```python
from build123d import *

# Parameters (mm, degrees)
F0_W      = 146.1516
F0_H      = 143.1798
F1_DEPTH  = 20.9042
F2_W      = 136.906
F2_H      = 134.874
F3_DEPTH  = 12.7
F4_W      = 13.97
F4_H      = 11.176
F5_DEPTH  = 12.7
F6_W      = 22.733
F6_H      = 6.096
F7_DEPTH  = 12.7
F8_W      = 15.367
F8_H      = 5.08
F9_DEPTH  = 12.7
F10_W     = 36.703
F10_H     = 12.319
F11_DEPTH = 12.7
F13_DEPTH = 12.7
F14_W     = 22.83968
F14_H     = 21.22805
F15_DEPTH = 12.7
F16_W     = 3.0399242607
F16_H     = 20.8479667597
F17_DEPTH = 12.7
F19_DEPTH = 12.7
F20_W     = 0.0204666441
F20_H     = 21.22805
F21_DEPTH = 12.7
F22_W     = 36.7188937962
F22_H     = 20.8685005598
F23_DEPTH = 12.7
F24_W     = 35.306
F24_H     = 13.2634267211
F25_DEPTH = 12.7
F27_DEPTH = 12.7
F28_W     = 1.4742958935
F28_H     = 20.8479667597
F29_DEPTH = 12.7
F30_W     = 0.2049181255
F30_H     = 13.2839605212
F31_DEPTH = 12.7
F32_W     = 50.9417812916
F32_H     = 3.8105603307
F33_DEPTH = 12.7
F34_W     = 0.1417576911
F34_H     = 9.2577636242
F35_DEPTH = 12.7
F36_W     = 44.7041876614
F36_H     = 0.2025440335
F37_DEPTH = 12.7
F38_W     = 8.9374343662
F38_H     = 3.9174016565
F39_DEPTH = 12.7
F40_W     = 127.9685656338
F40_H     = 2.8044246137
F41_DEPTH = 12.7
F42_W     = 120.384439826
F42_H     = 1.1129770428
F43_DEPTH = 12.7
F45_DEPTH = 12.7
F46_W     = 12.3281155104
F46_H     = 3.9624
F47_DEPTH = 12.7
F48_W     = 4.6508648958
F48_H     = 7.4722463233
F49_DEPTH = 12.7
F51_DEPTH = 12.7
F52_W     = 0.5965952
F52_H     = 1.6107708216
F53_DEPTH = 12.7
F55_DEPTH = 12.7
F57_DEPTH = 12.7
F58_DEPTH = 12.7
F59_W     = 18.6266698875
F59_H     = 19.8514753814
F60_DEPTH = 12.7
F61_W     = 2.536320244
F61_H     = 7.62
F62_DEPTH = 12.7


with BuildPart() as f1:
    # F0 (on Top) → F1 (new body)
    with BuildSketch(Plane.XY):
        Rectangle(F0_W, F0_H)
    extrude(amount=F1_DEPTH)

    # F2 (on face) → F3 (cut)
    with BuildSketch(Plane.XY.offset(20.9042)):
        Rectangle(F2_W, F2_H)
    extrude(amount=-F3_DEPTH, mode=Mode.SUBTRACT)

    # F4 (on face) → F5 (join)
    with BuildSketch(Plane.XY.offset(8.2042)):
        with Locations((-61.468, -61.849)):
            Rectangle(F4_W, F4_H)
    extrude(amount=F5_DEPTH)

    # F6 (on face) → F7 (join)
    with BuildSketch(Plane.XY.offset(8.2042)):
        with Locations((-43.1165, -59.309)):
            Rectangle(F6_W, F6_H)
    extrude(amount=F7_DEPTH)

    # F8 (on face) → F9 (join)
    with BuildSketch(Plane.XY.offset(8.2042)):
        with Locations((-39.4335, -64.897)):
            Rectangle(F8_W, F8_H)
    extrude(amount=F9_DEPTH)

    # F10 (on face) → F11 (join)
    with BuildSketch(Plane.XY.offset(8.2042)):
        with Locations((50.1015, -61.2775)):
            Rectangle(F10_W, F10_H)
    extrude(amount=F11_DEPTH)

    # F12 (on face) → F13 (join)
    with BuildSketch(Plane.XY.offset(8.2042)):
        Polygon((31.75, -56.261), (31.75, -55.118), (-60.8972720802, -55.118), (-60.8972720802, -56.261), (-31.75, -56.261), (-31.75, -59.817), (31.75, -59.817), (31.75, -57.820610702), align=None)
    extrude(amount=F13_DEPTH)

    # F14 (on face) → F15 (join)
    with BuildSketch(Plane.XY.offset(8.2042)):
        with Locations((-12.7041547344, -44.503975)):
            Rectangle(F14_W, F14_H)
    extrude(amount=F15_DEPTH)

    # F16 (on face) → F17 (join)
    with BuildSketch(Plane.XY.offset(8.2042)):
        with Locations((0.235647396, -44.6940166202)):
            Rectangle(F16_W, F16_H)
    extrude(amount=F17_DEPTH)

    # F18 (on face) → F19 (join)
    with BuildSketch(Plane.XY.offset(8.2042)):
        Polygon((24.1150483489, -33.88995), (1.2599385809, -33.88995), (1.2599385809, -34.2700332403), (1.7556095263, -34.2700332403), (1.7556095263, -55.118), (24.1150483489, -55.118), align=None)
    extrude(amount=F19_DEPTH)

    # F20 (on face) → F21 (join)
    with BuildSketch(Plane.XY.offset(8.2042)):
        with Locations((-24.1342280564, -44.503975)):
            Rectangle(F20_W, F20_H)
    extrude(amount=F21_DEPTH)

    # F22 (on face) → F23 (join)
    with BuildSketch(Plane.XY.offset(8.2042)):
        with Locations((42.474495247, -44.6837497201)):
            Rectangle(F22_W, F22_H)
    extrude(amount=F23_DEPTH)

    # F24 (on face) → F25 (join)
    with BuildSketch(Plane.XY.offset(8.2042)):
        with Locations((43.1809421451, -27.6177860796)):
            Rectangle(F24_W, F24_H)
    extrude(amount=F25_DEPTH)

    # F26 (on face) → F27 (join)
    with BuildSketch(Plane.XY.offset(8.2042)):
        Polygon((-25.618757272, -20.9860727191), (-60.924757272, -20.9860727191), (-60.924757272, -55.118), (-60.8972720802, -55.118), (-25.618757272, -55.118), align=None)
    extrude(amount=F27_DEPTH)

    # F28 (on face) → F29 (join)
    with BuildSketch(Plane.XY.offset(8.2042)):
        with Locations((-24.8816093252, -44.6940166202)):
            Rectangle(F28_W, F28_H)
    extrude(amount=F29_DEPTH)

    # F30 (on face) → F31 (join)
    with BuildSketch(Plane.XY.offset(8.2042)):
        with Locations((-25.5162982092, -27.6280529797)):
            Rectangle(F30_W, F30_H)
    extrude(amount=F31_DEPTH)

    # F32 (on face) → F33 (join)
    with BuildSketch(Plane.XY.offset(8.2042)):
        with Locations((0.0570514993, -22.8913528845)):
            Rectangle(F32_W, F32_H)
    extrude(amount=F33_DEPTH)

    # F34 (on face) → F35 (join)
    with BuildSketch(Plane.XY.offset(8.2042)):
        with Locations((25.4570632995, -29.6206176281)):
            Rectangle(F34_W, F34_H)
        Polygon((25.5279421451, -24.991735816), (25.5279421451, -24.7966330498), (21.3277284056, -24.7966330498), (21.3277284056, -24.991735816), (25.386184454, -24.991735816), align=None)
    extrude(amount=F35_DEPTH)

    # F36 (on face) → F37 (join)
    with BuildSketch(Plane.XY.offset(8.2042)):
        with Locations((-3.0617453158, -24.8979050666)):
            Rectangle(F36_W, F36_H)
    extrude(amount=F37_DEPTH)

    # F38 (on face) → F39 (join)
    with BuildSketch(Plane.XY.offset(8.2042)):
        with Locations((-63.9842828169, 21.8571154401)):
            Rectangle(F38_W, F38_H)
    extrude(amount=F39_DEPTH)

    # F40 (on face) → F41 (join)
    with BuildSketch(Plane.XY.offset(8.2042)):
        with Locations((4.4687171831, 22.4136039615)):
            Rectangle(F40_W, F40_H)
    extrude(amount=F41_DEPTH)

    # F42 (on face) → F43 (join)
    with BuildSketch(Plane.XY.offset(8.2042)):
        with Locations((0.6766542792, 20.4549031332)):
            Rectangle(F42_W, F42_H)
    extrude(amount=F43_DEPTH)

    # F44 (on face) → F45 (join)
    with BuildSketch(Plane.XY.offset(8.2042)):
        Polygon((-60.924757272, 19.8984146118), (-60.924757272, -20.9860727191), (60.8339421451, -20.9860727191), (60.8688741922, -20.9860727191), (60.8688741922, 19.8984146118), align=None)
    extrude(amount=F45_DEPTH)

    # F46 (on face) → F47 (join)
    with BuildSketch(Plane.XY.offset(8.2042)):
        with Locations((-62.2889422448, 33.2692625916)):
            Rectangle(F46_W, F46_H)
    extrude(amount=F47_DEPTH)

    # F48 (on face) → F49 (join)
    with BuildSketch(Plane.XY.offset(8.2042)):
        Polygon((-59.9482320249, 47.5855246186), (-56.1248844896, 47.5855246186), (-7.6236505993, 47.5855246186), (-7.6236505993, 67.437), (-68.453, 67.437), (-68.453, 55.3214401007), (-59.9482320249, 55.3214401007), align=None)
        Polygon((-58.2667700946, 42.6384061575), (-58.2667700946, 35.2504625916), (-56.1248844896, 35.2504625916), (-56.1248844896, 47.5855246186), (-59.9482320249, 47.5855246186), (-68.453, 47.5855246186), (-68.453, 42.6384061575), align=None)
        with Locations((-58.4503169375, 27.55193943)):
            Rectangle(F48_W, F48_H)
    extrude(amount=F49_DEPTH)

    # F50 (on face) → F51 (join)
    with BuildSketch(Plane.XY.offset(8.2042)):
        Polygon((13.3893499151, 66.3282424212), (13.3893499151, 66.38789922), (13.3893499151, 67.437), (11.0030192882, 67.437), (11.0030192882, 47.5855246186), (36.7157235742, 47.5855246186), (36.7157235742, 67.437), (29.7357104719, 67.437), (29.7357104719, 66.3282424212), (29.7357104719, 49.3256412446), (13.3893499151, 49.3256412446), (13.3893499151, 59.1095946729), (12.7927670255, 59.1095946729), (12.7927670255, 60.7203654945), (13.3893499151, 60.7203654945), align=None)
    extrude(amount=F51_DEPTH)

    # F52 (on face) → F53 (cut)
    with BuildSketch(Plane.XY.offset(20.9042)):
        with Locations((30.0340080719, 59.9149800837)):
            Rectangle(F52_W, F52_H)
    extrude(amount=-F53_DEPTH, mode=Mode.SUBTRACT)

    # F54 (on face) → F55 (join)
    with BuildSketch(Plane.XY.offset(8.2042)):
        Polygon((36.7157235742, 67.437), (36.7157235742, 61.2382255495), (36.7157235742, 47.5855246186), (36.7157235742, 44.6023866534), (68.453, 44.6733043295), (68.453, 67.437), align=None)
        Polygon((39.0854626894, 61.2382255495), (38.8847962022, 61.2382255495), (38.873040642, 63.3154974574), (39.0944701822, 63.3159922468), (39.0854626894, 67.3470505811), (48.391856432, 67.3678459326), (48.3948141336, 66.0442070147), (48.0193123221, 66.044986248), (48.0035748597, 58.4613198814), (48.376891034, 58.462154065), (48.3826112146, 55.9022428945), (48.0023957789, 55.9013932943), (48.0193123221, 48.3308546245), (48.3948141336, 48.3308546245), (48.3948141336, 47.008857131), (39.0854626894, 47.008857131), align=None, mode=Mode.SUBTRACT)
    extrude(amount=F55_DEPTH)

    # F56 (on face) → F57 (join)
    with BuildSketch(Plane.XY.offset(8.2042)):
        Polygon((-56.1248844896, 44.6023866534), (36.7157235742, 44.6023866534), (36.7157235742, 47.5855246186), (11.0030192882, 47.5855246186), (-7.6236505993, 47.5855246186), (-56.1248844896, 47.5855246186), align=None)
    extrude(amount=F57_DEPTH)

    # F58 (add): a face of the model
    f58_faces = [f1.faces().sort_by_distance(p)[0] for p in [
        (6.1865200926, 34.2136264879, 8.2042),
    ]]
    extrude(f58_faces, amount=F58_DEPTH)

    # F59 (on face) → F60 (join)
    with BuildSketch(Plane.XY.offset(8.2042)):
        with Locations((1.6896843445, 57.5112623093)):
            Rectangle(F59_W, F59_H)
        Polygon((-5.9129633009, 52.9398955405), (-5.9129633009, 54.9593605101), (-6.353115936, 54.9970567226), (-6.353115936, 56.5094996253), (-5.934735491, 56.5619803965), (-5.934735491, 61.7567235961), (-6.353115936, 61.8088580668), (-6.353115936, 63.3012766497), (-5.9279869311, 63.3546039462), (-5.9279869311, 65.3928667307), (-5.0910133868, 65.3928667307), (-5.0910133868, 66.3584321737), (-4.1863322258, 66.3584321737), (-4.1863322258, 66.9948086143), (7.1273995563, 66.9948086143), (7.1273995563, 66.3435682654), (8.0246776342, 66.3435682654), (8.0246776342, 65.3805136681), (8.8445162401, 65.3805136681), (8.8445162401, 63.3501261473), (9.2323757708, 63.3093193173), (9.2695318162, 63.2747858763), (9.2695318162, 61.8418827653), (9.2323757708, 61.8088580668), (8.8445162401, 61.7602057755), (8.8445162401, 56.5535761416), (9.1401832178, 56.5167330205), (9.2323757708, 56.4947389066), (9.2673106119, 56.4729869366), (9.2748431489, 56.4584843814), (9.2748431489, 55.0567209721), (9.2683695257, 55.0422929227), (9.234521538, 55.0210215151), (9.1941989958, 55.0067797303), (9.1401832178, 54.9970567226), (8.9794592932, 54.9773350358), (8.8445162401, 54.9603402615), (8.8445162401, 52.935667336), (8.0229612067, 52.935667336), (8.0229612067, 51.9765391946), (7.1176989004, 51.9765391946), (7.1176989004, 51.3154454529), (-4.1863322258, 51.3154454529), (-4.1863322258, 51.9765391946), (-5.0910133868, 51.9765391946), (-5.0910133868, 52.380554378), (-5.0910133868, 52.9398955405), align=None, mode=Mode.SUBTRACT)
    extrude(amount=F60_DEPTH)

    # F61 (on face) → F62 (join)
    with BuildSketch(Plane.XY.offset(8.2042)):
        with Locations((0.0027513015, -63.627)):
            Rectangle(F61_W, F61_H)
    extrude(amount=F62_DEPTH)


solid = f1.part
```
Work out the finished part from the listing and answer in its coordinate system (mm). Round coordinates to 2 decimals unless told otherwise and drop trailing zeros. Write each loop counter-clockwise with the first axis right and the second up, starting at its lowest first coordinate (ties: lowest second). Pieces come first, ordered by that corner, then holes. Notation, with made-up numbers: (-25.75, -33) -> (-2.75, -33) arc R34 cw to (-2.75, 3) -> close; hole circle Ø3 at (-20.75, 38.5). An arc over 180 degrees is marked (long way). Write each question's results on one line, items separated by ' | '.
1) The part is cut by section D-D (x = -28.5). Write down the section's boundary in (y, z), and give its area (3 significant figures).
Findings:
outline: (-71.59, 0) -> (71.59, 0) -> (71.59, 20.9) -> (-59.82, 20.9) -> (-59.82, 8.2) -> (-67.44, 8.2) -> (-67.44, 20.9) -> (-71.59, 20.9) -> close | area: 2,900 mm²
2) Consider line 1 along X through (y, z) = (49, 8.25); line 2 along Y through (x, z) = (-61.5, 13); line 3 along X through (y, z) = (51.5, 10.75). Determine where each line is inside the solid, lowest interval first. Write a range as [from, to].
Findings:
line 1: x = [-73.08, -68.45], [-59.95, 39.09], [48.02, 73.08] | line 2: y = [-71.59, -56.26], [19.9, 23.82], [31.29, 35.25], [42.64, 47.59], [55.32, 71.59] | line 3: x = [-73.08, -68.45], [-59.95, -4.19], [7.12, 13.39], [29.74, 39.09], [48.01, 73.08]
3) The part is cut by section A-A (x = -13.5). Write down the section's boundary in (y, z), and give its area (3 significant figures).
Findings:
outline: (-71.59, 0) -> (71.59, 0) -> (71.59, 20.9) -> (-25, 20.9) -> (-25, 8.2) -> (-33.89, 8.2) -> (-33.89, 20.9) -> (-59.82, 20.9) -> (-59.82, 8.2) -> (-67.44, 8.2) -> (-67.44, 20.9) -> (-71.59, 20.9) -> close | area: 2,780 mm²
4) For a pull along X with two mould halves and no side action, classify faces 1 (the flat face through (65, -17, 8.204)), 2 (the flat face through (-1, 1, 20.904)) as +X half, -X half, draft (parallel to the pull), parting line (faces both ways), or undercut.
Findings:
face 1: undercut | face 2: draft
5) A flat-ended cylindrical pin translates along its axis: pin 1 (8 mm diameter, centred on x = 20.5, y = -2.5, fed in from -Z). Find the tip coordinate at first contact, or state that the pin passes through.
Findings:
pin 1: stops at z = 0
6) The part is cut by section B-B (y = -51). Write down the section's boundary in (x, z), and give its area (3 significant figures).
Findings:
outline: (-73.08, 0) -> (73.08, 0) -> (73.08, 20.9) -> (68.45, 20.9) -> (68.45, 8.2) -> (60.83, 8.2) -> (60.83, 20.9) -> (-60.92, 20.9) -> (-60.92, 8.2) -> (-68.45, 8.2) -> (-68.45, 20.9) -> (-73.08, 20.9) -> close | area: 2,860 mm²
7) The part is cut by section C-C (z = 13.5). State how many separate pieces and enclosed holes the cut face has, and give its area (3 significant figures).
Findings:
separate pieces: 1 | enclosed holes: 12 | area: 17,900 mm²
